```python
from build123d import *

# Parameters (mm, degrees)
BOSS_EXTRUDE1_DEPTH        = 6.35
SKETCH2_R                  = 4.7625
CUT_EXTRUDE1_DEPTH         = 6.35
SKETCH3_R                  = 2.13995
CUT_EXTRUDE2_DEPTH         = 6.35
CUT_EXTRUDE4_DEPTH         = 6.35
F_6_32_TAPPED_HOLE1_REACH  = 59.727
F_6_32_TAPPED_HOLE1_BORE_R = 1.35255


with BuildPart() as part:
    # Sketch1 → Boss-Extrude1 (new body)
    with BuildSketch(Plane.XY):
        Polygon((-25.683252906, 38.866643011), (25.116747094, 38.866643011), (25.116747094, -6.027856989), (18.703247094, -6.027856989), (18.703247094, -12.441356989), (-19.269752906, -12.441356989), (-19.269752906, -6.027856989), (-25.683252906, -6.027856989), align=None)
    extrude(amount=BOSS_EXTRUDE1_DEPTH)

    # Sketch2 → Cut-Extrude1 (cut)
    with BuildSketch(Plane.XY.offset(6.35)):
        with Locations((-0.283252906, 26.103143011)):
            Circle(SKETCH2_R)
    extrude(amount=-CUT_EXTRUDE1_DEPTH, mode=Mode.SUBTRACT)

    # Sketch3 → Cut-Extrude2 (cut)
    with BuildSketch(Plane.XY.offset(6.35)):
        with Locations((-19.333252906, 29.341643011)):
            Circle(SKETCH3_R)
        with Locations((18.766747094, 29.341643011)):
            Circle(SKETCH3_R)
    extrude(amount=-CUT_EXTRUDE2_DEPTH, mode=Mode.SUBTRACT)

    # Sketch6 → Cut-Extrude4 (cut)
    with BuildSketch(Plane.XY.offset(6.35)):
        with BuildLine():
            Line((4.679797411, 8.060661082), (4.679797411, -1.058338959))
            ThreePointArc((4.679797411, -1.058338959), (-0.283252906, -6.021389275), (-5.246303222, -1.058338959))
            Line((-5.246303222, -1.058338959), (-5.246303222, 8.060661082))
            ThreePointArc((-5.246303222, 8.060661082), (-0.283252906, 13.023711398), (4.679797411, 8.060661082))
        make_face()
    extrude(amount=-CUT_EXTRUDE4_DEPTH, mode=Mode.SUBTRACT)

    # #6-32 Tapped Hole1 bore → #6-32 Tapped Hole1 (cut, up to next)
    with BuildSketch(Plane(origin=(0, 38.866643011, 0), x_dir=(1, 0, 0), z_dir=(0, 1, 0)), mode=Mode.PRIVATE) as f_6_32_tapped_hole1_sk1:
        with Locations((-0.283252906, -3.175)):
            Circle(F_6_32_TAPPED_HOLE1_BORE_R)
    f_6_32_tapped_hole1_tool1 = extrude(f_6_32_tapped_hole1_sk1.sketch, amount=-F_6_32_TAPPED_HOLE1_REACH, mode=Mode.PRIVATE) & part.part
    add(f_6_32_tapped_hole1_tool1.solids().sort_by_distance((-0.283253, 38.866643, 3.175))[0], mode=Mode.SUBTRACT)


solid = part.part
```
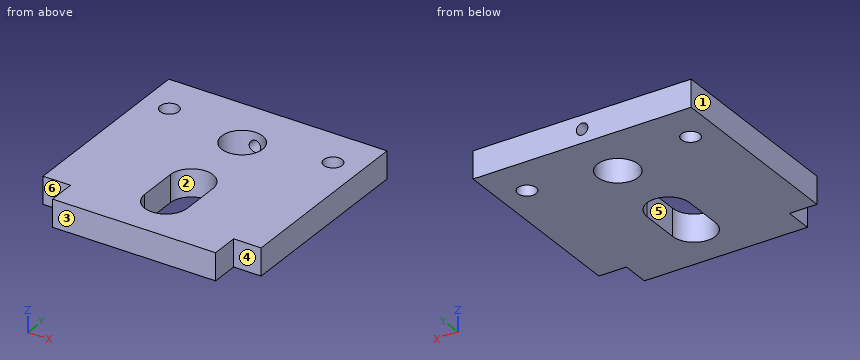
Work out the finished part from the listing and answer in its coordinate system (mm). Face numbers are marked on the shaded views. A direction names the side the tool comes from. Round coordinates to 2 decimals unless told otherwise and drop trailing zeros. Loops run counter-clockwise (first coordinate to the right, second up) from the corner with the lowest first, then second, coordinate; pieces in that order, holes last.
(1) The part is cut by section A-A, the plane y = 4. Give the vertices of the cut face in (x, z).
Computed values:
outline: (-25.68, 0) - (-5.25, 0) - (-5.25, 6.35) - (-25.68, 6.35) - close; (4.68, 0) - (25.12, 0) - (25.12, 6.35) - (4.68, 6.35) - close
(2) The part is cut by section D-D, the plane y = 34.5. Give the vertices of the cut face in (x, z) (3 decimals), and give its area (3 significant figures).
Computed values:
outline: (-25.683, 0) - (25.117, 0) - (25.117, 6.35) - (-25.683, 6.35) - close; hole circle Ø2.705 at (-0.283, 3.175)
area: 317 mm2
(3) Find the intervals of material crossed by L1, parallel to X at y = -2.5, z = 3.75; L2, parallel to X at y = 0, z = 3.75; L3, parallel to Y at x = 0, z = 5.25, in increasing order.
Computed values:
L1: x = -25.68 to -5.03, 4.47 to 25.12
L2: x = -25.68 to -5.25, 4.68 to 25.12
L3: y = -12.44 to -6.01, 13.02 to 21.35, 30.86 to 38.87
(4) The part is cut by section C-C, the plane x = 2. Give the vertices of the cut face in (y, z) (3 decimals).
Computed values:
outline: (-12.441, 0) - (-5.465, 0) - (-5.465, 6.35) - (-12.441, 6.35) - close; (12.467, 0) - (21.924, 0) - (21.924, 6.35) - (12.467, 6.35) - close; (30.283, 0) - (38.867, 0) - (38.867, 6.35) - (30.283, 6.35) - close
(5) Each of these flat-tipped pins is pushed along its axis until it touches: P1, Ø3, axis at x = -21, z = 3.5, coming from the -Y side; P2, Ø1.9, axis at y = -9, z = 1.5, coming from the -X side; P3, Ø11, axis at x = -0.28, y = 26.1, coming from the -Z side; P4, Ø2.5, axis at x = -0.28, z = 3.18, coming from the +Y side. Where does it stop, or does it pass through?
Computed values:
P1: stops at y = -6.03
P2: stops at x = -19.27
P3: stops at z = 0
P4: stops at y = 21.51
(6) For the marked faces 4, 5 and 6, determine the directions among +Z, -Z, +X, -X, +Y, -Y from which every point of the face is accessible in a straight line to the end or side of a thin tool.
Computed values:
face 4: +Z, -Z, +X, -Y
face 5: +Z, -Z
face 6: +Z, -Z, -X, -Y
(7) The mould has two halves that part along X. Classify the marked faces 1, 2 and 3: pulls with the +X half, pulls with the -X half, needs draft (parallel to the pull), parting line crosses it, or undercut.
Computed values:
face 1: pulls with the -X half
face 2: undercut
face 3: needs draft
(8) The part is cut by section B-B, the plane z = 5.5. Give the vertices of the cut face in (x, y) (1 decimal), and give its area (3 significant figures).
Computed values:
outline: (-25.7, -6) - (-19.3, -6) - (-19.3, -12.4) - (18.7, -12.4) - (18.7, -6) - (25.1, -6) - (25.1, 38.9) - (-25.7, 38.9) - close; hole circle Ø4.3 at (-19.3, 29.3); hole (-5.2, -1.1) arc R5 ccw to (4.7, -1.1) - (4.7, 8.1) arc R5 ccw to (-5.2, 8.1) - close; hole circle Ø9.5 at (-0.3, 26.1); hole circle Ø4.3 at (18.8, 29.3)
area: 2,260 mm2
